```python
from build123d import *

# Parameters (mm, degrees)
SKETCH_1_W      = 47.7
SKETCH_1_H      = 33.2
EXTRUDE_1_DEPTH = 10.2
SKETCH_2_R      = 0.5
EXTRUDE_2_DEPTH = 4
FILLET_1_R      = 1
FILLET_2_R      = 1
FILLET_3_R      = 1
FILLET_4_R      = 1


with BuildPart() as part:
    # Эскиз1 → Бобышка-Вытянуть1 (new body)
    with BuildSketch(Plane(origin=(0, 0, 0), x_dir=(1, 0, 0), z_dir=(0, 1, 0))):
        Rectangle(SKETCH_1_W, SKETCH_1_H)
    extrude(amount=EXTRUDE_1_DEPTH)

    # Эскиз2 → Бобышка-Вытянуть2 (add)
    with BuildSketch(Plane(origin=(0, 10.2, 0), x_dir=(1, 0, 0), z_dir=(0, 1, 0))):
        with Locations(Location((-20.85, 5.9, 0), (0, 0, 270))):
            Circle(SKETCH_2_R)
        with Locations(Location((-20.85, 10.9, 0), (0, 0, 270))):
            Circle(SKETCH_2_R)
        with Locations(Location((-20.85, -12.85, 0), (0, 0, 270))):
            Circle(SKETCH_2_R)
        with Locations(Location((-20.85, -9.1, 0), (0, 0, 270))):
            Circle(SKETCH_2_R)
        with Locations(Location((20.9, -12.85, 0), (0, 0, 270))):
            Circle(SKETCH_2_R)
        with Locations(Location((20.9, -0.35, 0), (0, 0, 270))):
            Circle(SKETCH_2_R)
        with Locations(Location((20.9, 4.65, 0), (0, 0, 270))):
            Circle(SKETCH_2_R)
    extrude(amount=EXTRUDE_2_DEPTH)

    # Скругление1
    fillet_1_edges = [part.edges().sort_by_distance(p)[0] for p in [
        (0, 0, 16.6),
        (-23.85, 0, 0),
    ]]
    fillet(fillet_1_edges, radius=FILLET_1_R)

    # Скругление2
    fillet_2_edges = [part.edges().sort_by_distance(p)[0] for p in [
        (23.85, 0, -0.5),
        (-23.557106781, 0.292893219, -16.6),
        (23.85, 0.292893219, 16.307106781),
        (0.5, 0, -16.6),
        (23.85, 5.6, 16.6),
        (-23.85, 5.6, -16.6),
    ]]
    fillet(fillet_2_edges, radius=FILLET_2_R)

    # Скругление3
    # the kernel refuses this fillet: 1 mm, written as the material it takes off along each edge
    with BuildSketch(Plane(origin=(-22.85, 1, 15.6), x_dir=(0, 0, 1), z_dir=(-1, 0, 0))) as fillet_3_piece_1_section:
        Polygon((0, 0), (FILLET_3_R, 0), (FILLET_3_R, -FILLET_3_R), (0, -FILLET_3_R), align=None)
    fillet_3_piece_1 = extrude(amount=FILLET_3_R, mode=Mode.PRIVATE)
    fillet_3_piece_1 = fillet_3_piece_1 - Plane(origin=(-22.85, 1, 15.6), x_dir=(0, 0.7071067811865475, -0.7071067811865475), z_dir=(-1, 0, 0)) * Sphere(FILLET_3_R, mode=Mode.PRIVATE)
    add(fillet_3_piece_1, mode=Mode.SUBTRACT)
    with BuildSketch(Plane(origin=(-22.85, 9.2, 15.6), x_dir=(-1, 0, 0), z_dir=(0, 1, 0))) as fillet_3_piece_2_section:
        Polygon((0, 0), (FILLET_3_R, 0), (FILLET_3_R, FILLET_3_R), (0, FILLET_3_R), align=None)
    fillet_3_piece_2 = extrude(amount=FILLET_3_R, mode=Mode.PRIVATE)
    fillet_3_piece_2 = fillet_3_piece_2 - Plane(origin=(-22.85, 9.2, 15.6), x_dir=(0.7071067811865475, 0, -0.7071067811865475), z_dir=(0, 1, 0)) * Sphere(FILLET_3_R, mode=Mode.PRIVATE)
    add(fillet_3_piece_2, mode=Mode.SUBTRACT)
    with BuildSketch(Plane(origin=(22.85, 10.2, 16.6), x_dir=(0, 0, -1), z_dir=(-1, 0, 0))) as fillet_3_piece_3:
        with BuildLine():
            CenterArc((FILLET_3_R, FILLET_3_R), FILLET_3_R, 180, 90)
            Line((0, FILLET_3_R), (0, 0))
            Line((0, 0), (FILLET_3_R, 0))
        make_face()
    extrude(amount=45.7, mode=Mode.SUBTRACT)
    with BuildSketch(Plane(origin=(23.85, 10.2, -19.1), x_dir=(-1, 0, 0), z_dir=(0, 0, 1))) as fillet_3_piece_4:
        with BuildLine():
            CenterArc((FILLET_3_R, FILLET_3_R), FILLET_3_R, 180, 90)
            Line((0, FILLET_3_R), (0, 0))
            Line((0, 0), (FILLET_3_R, 0))
        make_face()
    extrude(amount=34.7, mode=Mode.SUBTRACT)
    with BuildSketch(Plane(origin=(-23.85, 10.2, 15.6), x_dir=(1, 0, 0), z_dir=(0, 0, -1))) as fillet_3_piece_5:
        with BuildLine():
            CenterArc((FILLET_3_R, FILLET_3_R), FILLET_3_R, 180, 90)
            Line((0, FILLET_3_R), (0, 0))
            Line((0, 0), (FILLET_3_R, 0))
        make_face()
    extrude(amount=31.2, mode=Mode.SUBTRACT)
    with BuildSketch(Plane(origin=(-22.85, 10.2, -15.6), x_dir=(0, 0, -1), z_dir=(1, 0, 0))) as fillet_3_piece_6:
        with BuildLine():
            CenterArc((1 - FILLET_3_R, -FILLET_3_R), FILLET_3_R, 0, 90)
            Line((1, -FILLET_3_R), (1, 0))
            Line((1, 0), (1 - FILLET_3_R, 0))
        make_face()
    revolve(axis=Axis((-22.85, 10.2, -15.6), (0, 1, 0)), revolution_arc=90, mode=Mode.SUBTRACT)
    with BuildSketch(Plane(origin=(22.85, 10.2, 15.6), x_dir=(0, 0, 1), z_dir=(-1, 0, 0))) as fillet_3_piece_7:
        with BuildLine():
            CenterArc((1 - FILLET_3_R, -FILLET_3_R), FILLET_3_R, 0, 90)
            Line((1, -FILLET_3_R), (1, 0))
            Line((1, 0), (1 - FILLET_3_R, 0))
        make_face()
    revolve(axis=Axis((22.85, 10.2, 15.6), (0, 1, 0)), revolution_arc=90, mode=Mode.SUBTRACT)
    with BuildSketch(Plane(origin=(-22.85, 10.2, -16.6), x_dir=(0, -1, 0), z_dir=(1, 0, 0))) as fillet_3_piece_8:
        with BuildLine():
            CenterArc((FILLET_3_R, -FILLET_3_R), FILLET_3_R, 90, 90)
            Line((0, -FILLET_3_R), (0, 0))
            Line((0, 0), (FILLET_3_R, 0))
        make_face()
    extrude(amount=49.2, mode=Mode.SUBTRACT)
    with BuildSketch(Plane(origin=(-23.85, 1, 16.6), x_dir=(0, 0, -1), z_dir=(0, 1, 0))) as fillet_3_piece_9:
        with BuildLine():
            CenterArc((FILLET_3_R, -FILLET_3_R), FILLET_3_R, 90, 90)
            Line((0, -FILLET_3_R), (0, 0))
            Line((0, 0), (FILLET_3_R, 0))
        make_face()
    extrude(amount=8.2, mode=Mode.SUBTRACT)

    # Скругление4
    # the kernel refuses this fillet: 1 mm, written as the material it takes off along each edge
    with BuildSketch(Plane(origin=(22.85, 1, -15.6), x_dir=(1, 0, 0), z_dir=(0, 0, -1))) as fillet_4_piece_1_section:
        Polygon((0, 0), (FILLET_4_R, 0), (FILLET_4_R, FILLET_4_R), (0, FILLET_4_R), align=None)
    fillet_4_piece_1 = extrude(amount=FILLET_4_R, mode=Mode.PRIVATE)
    fillet_4_piece_1 = fillet_4_piece_1 - Plane(origin=(22.85, 1, -15.6), x_dir=(-0.7071067811865475, 0.7071067811865475, 0), z_dir=(0, 0, -1)) * Sphere(FILLET_4_R, mode=Mode.PRIVATE)
    add(fillet_4_piece_1, mode=Mode.SUBTRACT)
    with BuildSketch(Plane(origin=(22.85, 9.2, -15.6), x_dir=(1, 0, 0), z_dir=(0, 0, -1))) as fillet_4_piece_2_section:
        Polygon((0, 0), (FILLET_4_R, 0), (FILLET_4_R, -FILLET_4_R), (0, -FILLET_4_R), align=None)
    fillet_4_piece_2 = extrude(amount=FILLET_4_R, mode=Mode.PRIVATE)
    fillet_4_piece_2 = fillet_4_piece_2 - Plane(origin=(22.85, 9.2, -15.6), x_dir=(-0.7071067811865475, -0.7071067811865475, 0), z_dir=(0, 0, -1)) * Sphere(FILLET_4_R, mode=Mode.PRIVATE)
    add(fillet_4_piece_2, mode=Mode.SUBTRACT)
    with BuildSketch(Plane(origin=(23.85, 1, -16.6), x_dir=(-1, 0, 0), z_dir=(0, 1, 0))) as fillet_4_piece_3:
        with BuildLine():
            CenterArc((FILLET_4_R, FILLET_4_R), FILLET_4_R, 180, 90)
            Line((0, FILLET_4_R), (0, 0))
            Line((0, 0), (FILLET_4_R, 0))
        make_face()
    extrude(amount=8.2, mode=Mode.SUBTRACT)


solid = part.part
```
For this review, take the finished solid that the model builds, in its own axes (mm). A direction names the side the tool comes from. Coordinates: 2 decimals unless noted, no trailing zeros. Loops run counter-clockwise (first coordinate to the right, second up) from the corner with the lowest first, then second, coordinate; pieces in that order, holes last.
1. Insertion check: P1, Ø8, axis at x = 3, z = -2.5, coming from the +Y side; P2, Ø8, axis at x = -12, y = 10, coming from the -Z side. Each pin has a flat end and moves straight along its axis. Give the tip position at first contact, or say it passes through.
2. Add section C-C, the plane z = -4.65. Give the boundary of the cut face in (x, y), then the cut area to 3 significant figures.
3. Add section A-A, the plane y = 12.5. Give the boundary of the cut face in (x, z).
4. Add section B-B, the plane x = 20.9. Give the boundary of the cut face in (y, z).
5. Add section D-D, the plane x = 3. Give the boundary of the cut face in (y, z), then the cut area to 3 significant figures.
6. For faces 4 (the cylindrical face through (0.32, 0.301, 16.315)), 5 (the cylindrical face through (-21.338, 12.172, -11.008)), list the 3-axis set-ups (+Z, -Z, +X, -X, +Y, -Y) from which the entire face can be reached by the end or side of a thin tool; tool diameter is ignored.
7. For line 1 (Y direction, x = 10, z = -3); line 2 (X direction, y = 9.5, z = -9), list the stretches that pass through material, from the lowest coordinate up.
8. Mouldability with a two-part tool opening along Z and no side actions: class faces 1 (the flat face through (20.9, 14.2, -4.7)), 2 (the cylindrical face through (-21.338, 12.172, -6.008)), 3 (the cylindrical face through (-0.32, 9.899, -16.315)) as +Z half, -Z half, draft (parallel to the pull), parting line (faces both ways), or undercut.
Result:
1. P1: stops at y = 10.2
1. P2: stops at z = -16.6
2. outline: (-23.85, 1) arc R1 ccw to (-22.85, 0) - (22.85, 0) arc R1 ccw to (23.85, 1) - (23.85, 9.2) arc R1 ccw to (22.85, 10.2) - (21.4, 10.2) - (21.4, 14.2) - (20.4, 14.2) - (20.4, 10.2) - (-22.85, 10.2) arc R1 ccw to (-23.85, 9.2) - close
2. area: 490 mm2
3. outline: circle Ø1 at (-20.85, -10.9); circle Ø1 at (-20.85, -5.9); circle Ø1 at (-20.85, 9.1); circle Ø1 at (-20.85, 12.85); circle Ø1 at (20.9, -4.65); circle Ø1 at (20.9, 0.35); circle Ø1 at (20.9, 12.85)
4. outline: (0, -15.6) arc R1 ccw to (1, -16.6) - (9.2, -16.6) arc R1 ccw to (10.2, -15.6) - (10.2, -5.15) - (14.2, -5.15) - (14.2, -4.15) - (10.2, -4.15) - (10.2, -0.15) - (14.2, -0.15) - (14.2, 0.85) - (10.2, 0.85) - (10.2, 12.35) - (14.2, 12.35) - (14.2, 13.35) - (10.2, 13.35) - (10.2, 15.6) arc R1 ccw to (9.2, 16.6) - (1, 16.6) arc R1 ccw to (0, 15.6) - close
5. outline: (0, -15.6) arc R1 ccw to (1, -16.6) - (9.2, -16.6) arc R1 ccw to (10.2, -15.6) - (10.2, 15.6) arc R1 ccw to (9.2, 16.6) - (1, 16.6) arc R1 ccw to (0, 15.6) - close
5. area: 338 mm2
6. face 4: +Z, +X, -X, -Y
6. face 5: +Y
7. line 1: y = 0 to 10.2
7. line 2: x = -23.8 to 23.8
8. face 1: draft
8. face 2: undercut
8. face 3: -Z half
